```python
from build123d import *

# Parameters (mm, degrees)
F2_R     = 10
F3_DEPTH = 50


with BuildPart() as f1:
    # F0 (on Top) → F1 (revolve)
    with BuildSketch(Plane.XY):
        Polygon((15, -15), (25, -15), (25, 15), (-25, 15), (-25, -15), (-15, -15), (-15, -5), (-5, -5), (-5, -15), (5, -15), (5, -5), (15, -5), align=None)
    revolve(axis=Axis((0, 15, 0), (-1, 0, 0)))

    # F2 (on face) → F3 (cut)
    with BuildSketch(Plane.YZ.offset(25)):
        with Locations((15, 0)):
            Circle(F2_R)
    extrude(amount=-F3_DEPTH, mode=Mode.SUBTRACT)


solid = f1.part
```
For this review, take the finished solid that the model builds, in its own axes (mm). A direction names the side the tool comes from. Coordinates: 2 decimals unless noted, no trailing zeros. Write each loop counter-clockwise with the first axis right and the second up, starting at its lowest first coordinate (ties: lowest second). Pieces come first, ordered by that corner, then holes.
(1) The part is to be moulded in two halves that separate along Y. For faces 3 (the face through (-15, -5, -6)), 4 (the face through (20, 39, -18)), 5 (the face through (0.35, 24.54, 3)), say which applies: +Y half, -Y half, draft (parallel to the pull), parting line (faces both ways), or undercut.
(2) Add section A-A on y = 15. Give the boundary of the cut face in (x, z), then the cut area to 3 significant figures.
(3) Wall thickness on probe 1 along X at (y, z) = (-7, -7); probe 2 along Z at (x, y) = (-6, 15); probe 3 along Z at (x, y) = (-14.5, 17): over which ranges is each line inside the solid? List them lowest first.
(4) For pin 1 Ø6 at (x, z) = (-0.5, 13.5) entering from -Y; pin 2 Ø1 at (x, z) = (4.5, 3.5) entering from +Y; pin 3 Ø8 at (x, z) = (14.5, 16) entering from +Y, all flat-tipped, find the tip position at first contact; note any pin that passes through.
(5) Add section B-B on z = 0. Give the boundary of the cut face in (x, y), then the cut area to 3 significant figures.
(6) Add section C-C on x = -18.5. Give the boundary of the cut face in (y, z).
(7) Tool access review of faces 1 (the face through (-20, 39, -18)), 2 (the face through (15, 21, -20)): name each direction out of +Z, -Z, +X, -X, +Y, -Y from which nothing blocks a thin tool from reaching the whole face with its end or side.
(8) Add section D-D on y = 4. Give the boundary of the cut face in (x, z).
Answer sheet:
1. face 3: draft
1. face 4: parting line
1. face 5: undercut
2. outline: (-25, -30) - (-15, -30) - (-15, -20) - (-5, -20) - (-5, -30) - (5, -30) - (5, -20) - (15, -20) - (15, -30) - (25, -30) - (25, -10) - (-25, -10) - close; (-25, 10) - (25, 10) - (25, 30) - (15, 30) - (15, 20) - (5, 20) - (5, 30) - (-5, 30) - (-5, 20) - (-15, 20) - (-15, 30) - (-25, 30) - close
2. area: 1,600 mm2
3. probe 1: x = -25 to -15, -5 to 5, 15 to 25
3. probe 2: z = -20 to -10, 10 to 20
3. probe 3: z = -19.9 to -9.8, 9.8 to 19.9
4. pin 1: stops at y = -13.1
4. pin 2: stops at y = 44.85
4. pin 3: stops at y = 42.48
5. outline: (-25, -15) - (-15, -15) - (-15, -5) - (-5, -5) - (-5, -15) - (5, -15) - (5, -5) - (15, -5) - (15, -15) - (25, -15) - (25, 5) - (-25, 5) - close; (-25, 25) - (25, 25) - (25, 45) - (15, 45) - (15, 35) - (5, 35) - (5, 45) - (-5, 45) - (-5, 35) - (-15, 35) - (-15, 45) - (-25, 45) - close
5. area: 1,600 mm2
6. outline: circle Ø60 at (15, 0); hole circle Ø20 at (15, 0)
7. face 1: +X, -X
7. face 2: none
8. outline: (-25, -27.91) - (-15, -27.91) - (-15, -16.7) - (-5, -16.7) - (-5, -27.91) - (5, -27.91) - (5, -16.7) - (15, -16.7) - (15, -27.91) - (25, -27.91) - (25, 27.91) - (15, 27.91) - (15, 16.7) - (5, 16.7) - (5, 27.91) - (-5, 27.91) - (-5, 16.7) - (-15, 16.7) - (-15, 27.91) - (-25, 27.91) - close
